The model under review builds one solid part; all positions refer to its coordinate system, in mm. A direction names the side the tool comes from. Give positions to 0.01 mm unless a question says otherwise; leave off trailing zeros. Order: outer loops, then holes, each group sorted by start corner. A loop starts at its lowest first (then second) coordinate and runs counter-clockwise, first axis right, second up.
```python
from build123d import *

# Parameters (mm, degrees)
PAD_DEPTH             = 14
SKETCH001_R           = 23
POCKET_DEPTH          = 10
SKETCH002_R           = 2.5
SKETCH002_R_2         = 1.5
POCKET001_DEPTH       = 173.2109287867
POLARPATTERN_COUNT    = 5
PAD001_DEPTH          = 21
POLARPATTERN001_COUNT = 8
SKETCH004_R           = 6.5
POCKET002_DEPTH       = 5
POLARPATTERN002_COUNT = 8


with BuildPart() as part:
    # Sketch → Pad (new body)
    with BuildSketch(Plane.XY):
        Polygon((29.5, 0), (20.859650045, 20.859650045), (0, 29.5), (-20.859650045, 20.859650045), (-29.5, 0), (-20.859650045, -20.859650045), (0, -29.5), (20.859650045, -20.859650045), align=None)
    extrude(amount=PAD_DEPTH)

    # Sketch001 (on Face10 of Pad) → Pocket (cut)
    with BuildSketch(Plane.XY.offset(14)):
        Circle(SKETCH001_R)
    extrude(amount=-POCKET_DEPTH, mode=Mode.SUBTRACT)

    # Sketch002 (on Face12 of Pocket) → Pocket001 (cut, through all)
    with BuildSketch(Plane.XY.offset(4)):
        Circle(SKETCH002_R)
        with Locations((0, 13.3)):
            Circle(SKETCH002_R_2)
    pocket001 = extrude(amount=-POCKET001_DEPTH, mode=Mode.SUBTRACT)

    # PolarPattern: Pocket001 ×5 about axis
    polarpattern_axis = Axis((0, 0, 4), (0, 0, 1))
    for i in range(1, POLARPATTERN_COUNT):
        add(pocket001.rotate(polarpattern_axis, i * 360 / POLARPATTERN_COUNT), mode=Mode.SUBTRACT)

    # Sketch003 (on Face8 of PolarPattern) → Pad001 (join)
    with BuildSketch(Plane(origin=(-10.4298250225, -25.1798250225, 0), x_dir=(0.9238795325, -0.3826834324, 0), z_dir=(-0.3826834324, -0.9238795325, 0))):
        Polygon((-11.2891612548, 14), (3.9092426218, 0), (11.2891612548, 0), (-3.9092426218, 14), align=None)
    pad001 = extrude(amount=PAD001_DEPTH)

    # PolarPattern001: Pad001 ×8 about axis
    polarpattern001_axis = Axis((0, 0, 0), (0, 0, 1))
    for i in range(1, POLARPATTERN001_COUNT):
        add(pad001.rotate(polarpattern001_axis, i * 360 / POLARPATTERN001_COUNT))

    # Sketch004 (on Face52 of PolarPattern001) → Pocket002 (cut)
    with BuildSketch(Plane(origin=(4.7875561885, -1.9830707039, 5.6255952654), x_dir=(0.7798699787, 0.208098843, -0.5903369274), z_dir=(0.6259415438, -0.2592734767, 0.7355096519))):
        with Locations((-21.9449518208, -32.1188270446)):
            Circle(SKETCH004_R)
        with BuildLine():
            Line((-14.1030025385, -36.5351412832), (-10.8005808993, -36.0996031065))
            Line((-10.8005808993, -36.0996031065), (-16.4436490931, -46.1198716338))
            Line((-16.4436490931, -46.1198716338), (-39.1781340839, -33.3165970703))
            Line((-33.5350658901, -23.296328543), (-39.1781340839, -33.3165970703))
            Line((-29.786901103, -27.7025128059), (-33.5350658901, -23.296328543))
            ThreePointArc((-29.786901103, -27.7025128059), (-26.3612660594, -39.9607763268), (-14.1030025385, -36.5351412832))
        make_face()
    pocket002 = extrude(amount=-POCKET002_DEPTH, mode=Mode.SUBTRACT)

    # PolarPattern002: Pocket002 ×8 about axis
    polarpattern002_axis = Axis((0, 0, 0), (0, 0, 1))
    for i in range(1, POLARPATTERN002_COUNT):
        add(pocket002.rotate(polarpattern002_axis, i * 360 / POLARPATTERN002_COUNT), mode=Mode.SUBTRACT)


solid = part.part
```
1. For faces 1 (the flat face through (17.62, -28.21, 5.35)), 2 (the flat face through (-3.999, -27.844, 10.013)), 3 (the flat face through (23.26, -31.49, 0.43)), 4 (the flat face through (-27.28, -5.36, 5.35)), 5 (the flat face through (-30.31, 18.49, 8.65)), list the 3-axis set-ups (+Z, -Z, +X, -X, +Y, -Y) from which the entire face can be reached by the end or side of a thin tool; tool diameter is ignored.
2. Insertion check: pin 1 (5 mm diameter, centred on y = -29.5, z = 10, fed in from +X); pin 2 (1.5 mm diameter, centred on y = -30.5, z = 10, fed in from -X); pin 3 (3 mm diameter, centred on x = 12.5, z = 11.5, fed in from -Y). Each pin has a flat end and moves straight along its axis. Give the tip position at first contact, or say it passes through.
3. Take a section at A-A (y = -5). Write out the cut boundary in (x, z), and give its area (3 significant figures).
4. To check wall thickness, follow line 1 (Y direction, x = -31.5, z = 8.75); line 2 (Y direction, x = -3.5, z = 8); line 3 (X direction, y = -12, z = 7.75). State the ranges of each line that lie inside material, in increasing order.
5. Take a section at B-B (z = 7.75). Count the separate pieces of the cut face and the enclosed holes in it, and give its area (3 significant figures).
Answer:
1. face 1: +Z, +X
1. face 2: +Z, -Y
1. face 3: -Z, +X
1. face 4: -Z, -X
1. face 5: -Z, +Y
2. pin 1: stops at x = 15.11
2. pin 2: stops at x = -21.09
2. pin 3: stops at y = -43.02
3. outline: (-38.37, 12.87) - (-27.43, 9.01) - (-27.43, 0) - (38.43, 0) - (38.86, 0.96) - (27.43, 4.99) - (27.43, 14) - (22.45, 14) - (22.45, 4) - (-22.45, 4) - (-22.45, 14) - (-38.1, 14) - close
3. area: 386 mm2
4. line 1: y = -11.33 to -7, 17.9 to 19.1
4. line 2: y = -28.05 to -22.73, 22.73 to 28.05
4. line 3: x = -30.39 to -19.62, 19.62 to 30.15
5. separate pieces: 9
5. enclosed holes: 1
5. area: 1,300 mm2
